Source: CAD feature listing. Evaluate the final solid. Frame: model axes, mm. Round coordinates to 2 decimals unless told otherwise and drop trailing zeros. Loops run counter-clockwise (first coordinate to the right, second up) from the corner with the lowest first, then second, coordinate; pieces in that order, holes last.
(1) Section A-A, the plane y = -4.5. Return the cut outline in (x, z).
(2) Section B-B, the plane z = 0. Return the cut outline in (x, y).
(3) First-contact query: pin 1 Ø2 at (y, z) = (-2, -5) entering from -X; pin 2 Ø1.5 at (x, z) = (0.5, 2) entering from -Y; pin 3 Ø6 at (x, y) = (-1.5, -15) entering from +Z. Flat tips, straight axial feed; report the tip coordinate or a pass-through.
(4) Mould query, pull axis X, two halves, no side actions, for faces 1 (the flat face through (2, 0, 2)), 2 (the flat face through (-2, -5, 3)), 3 (the cylindrical face through (7.493, -4.816, -0.33)), 4 (the cylindrical face through (0, -1, -2)). Classes: pulls with the +X half, pulls with the -X half, needs draft (parallel to the pull), parting line crosses it, or undercut.
(5) Section C-C, the plane x = 1. Return the cut outline in (y, z).
(6) Section D-D, the plane z = -3.25. Return the cut outline in (x, y), plus the area to 3 significant figures.
(7) Material intervals for probe 1 along Z at (x, y) = (0, -2.2); probe 2 along Y at (x, z) = (-1.25, 3.25); probe 3 along Y at (x, z) = (0.75, -2), sorted ascending.
```python
from build123d import *

# Parameters (mm, degrees)
CUT_EXTRUDE1_START = -3
CUT_EXTRUDE1_DEPTH = 3.5
CUT_EXTRUDE2_REACH = 22.037
SKETCH3_R          = 2


with BuildPart() as part:
    # Sketch1 → Revolve1 (revolve)
    with BuildSketch(Plane.XY):
        with BuildLine():
            Line((0, 0), (-7.5, 0))
            Line((-7.5, 0), (-7.5, -9.5))
            ThreePointArc((-7.5, -9.5), (-5.303300859, -14.803300859), (0, -17))
            Line((0, -17), (0, 0))
        make_face()
    revolve(axis=Axis((0, 0, 0), (0, -1, 0)))

    # Sketch2 → Cut-Extrude1 (cut)
    with BuildSketch(Plane(origin=(0, 0, 0), x_dir=(1, 0, 0), z_dir=(0, 1, 0)).offset(CUT_EXTRUDE1_START)):
        Polygon((3.6, -2.078460969), (3.6, 2.078460969), (0, 4.156921938), (-3.6, 2.078460969), (-3.6, -2.078460969), (0, -4.156921938), align=None)
    extrude(amount=-CUT_EXTRUDE1_DEPTH, mode=Mode.SUBTRACT)

    # Sketch3 → Cut-Extrude2 (cut, up to next)
    with BuildSketch(Plane(origin=(0, 0, 0), x_dir=(1, 0, 0), z_dir=(0, 1, 0)), mode=Mode.PRIVATE) as cut_extrude2_sk1:
        with Locations(Location((0, 0, 0), (0, 0, 180))):
            Circle(SKETCH3_R)
    cut_extrude2_tool1 = extrude(cut_extrude2_sk1.sketch, amount=-CUT_EXTRUDE2_REACH, mode=Mode.PRIVATE) & part.part
    add(cut_extrude2_tool1.solids().sort_by_distance((0, 0, 0))[0], mode=Mode.SUBTRACT)


solid = part.part
```
Output values:
1. outline: circle Ø15 at (0, 0); hole (-3.6, -2.08) - (0, -4.16) - (3.6, -2.08) - (3.6, 2.08) - (0, 4.16) - (-3.6, 2.08) - close
2. outline: (-7.5, -9.5) arc R7.5 ccw to (7.5, -9.5) - (7.5, 0) - (2, 0) - (2, -3) - (3.6, -3) - (3.6, -6.5) - (-3.6, -6.5) - (-3.6, -3) - (-2, -3) - (-2, 0) - (-7.5, 0) - close
3. pin 1: stops at x = -6.34
3. pin 2: stops at y = -16.88
3. pin 3: stops at z = 7
4. face 1: needs draft
4. face 2: undercut
4. face 3: parting line crosses it
4. face 4: undercut
5. outline: (-9.5, -7.43) - (0, -7.43) - (0, -1.73) - (-3, -1.73) - (-3, -3.58) - (-6.5, -3.58) - (-6.5, 3.58) - (-3, 3.58) - (-3, 1.73) - (0, 1.73) - (0, 7.43) - (-9.5, 7.43) arc R7.43 ccw to start
6. outline: (-6.76, -9.5) arc R6.76 ccw to (6.76, -9.5) - (6.76, 0) - (-6.76, 0) - close; hole (-1.57, -6.5) - (1.57, -6.5) - (1.57, -3) - (-1.57, -3) - close
6. area: 189 mm2
7. probe 1: z = -7.5 to -2, 2 to 7.5
7. probe 2: y = -16.14 to -6.5, -3 to 0
7. probe 3: y = -16.69 to -6.5, -3 to 0
